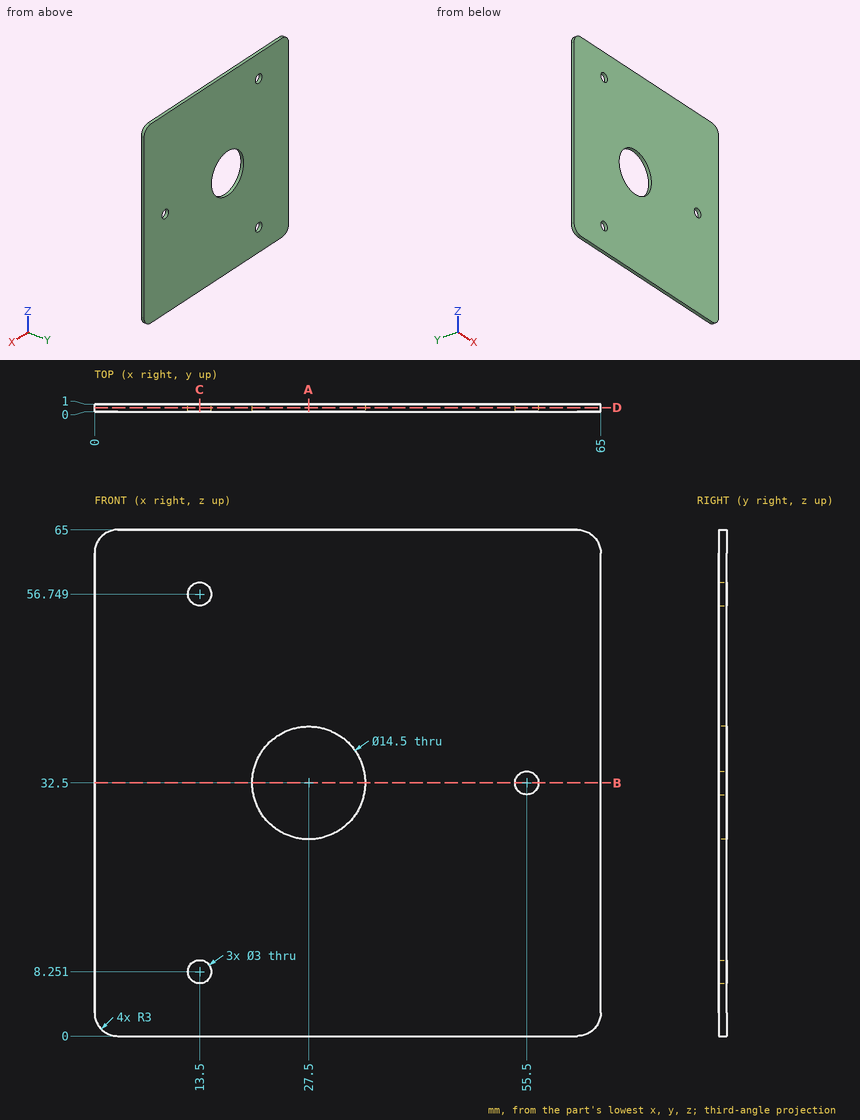
Geometry check sheet. Reference: drawing and pictorial views, mm from the part's lowest x, y, z. Give positions to 0.01 mm unless a question says otherwise; leave off trailing zeros. Loops run counter-clockwise (first coordinate to the right, second up) from the corner with the lowest first, then second, coordinate; pieces in that order, holes last. Notation, with made-up numbers: (-17, 46.5) - (-7, 46.5) arc R15 ccw to (-7, 74.5) - close; hole circle Ø5 at (28.5, -20.75). An arc over 180 degrees is marked (long way). Use CSV: the item, a comma, the result in double quotes. Start each with the question number.
Q1. Section check D-D, the plane y = 0.55. Record the cut outline in (x, z).
Q2. Section check C-C, the plane x = 13.5. Record the cut outline in (y, z).
Q3. Section check B-B, the plane z = 32.5. Record the cut outline in (x, y).
Q4. Scan lines: probe 1 along Z at (x, y) = (27, 0.4); probe 2 along X at (y, z) = (0.7, 33) (1 decimal); probe 3 along Z at (x, y) = (32, 0.65) (1 decimal). Record each from-to range of solid material in increasing order. Write a range as from..to.
Q5. Section check A-A, the plane x = 27.5. Record the cut outline in (y, z).
Q6. Go/stop test with a flat-tipped pin: pin 1 Ø8.5 at (x, z) = (27.5, 32.5) entering from -Y. Record where the tip stops, or that it passes through.
Findings below:
1,outline,"(0, 3) arc R3 ccw to (3, 0) - (62, 0) arc R3 ccw to (65, 3) - (65, 62) arc R3 ccw to (62, 65) - (3, 65) arc R3 ccw to (0, 62) - close; hole circle Ø3 at (13.5, 8.25); hole circle Ø3 at (13.5, 56.75); hole circle Ø14.5 at (27.5, 32.5); hole circle Ø3 at (55.5, 32.5)"
2,outline,"(0, 0) - (1, 0) - (1, 6.75) - (0, 6.75) - close; (0, 9.75) - (1, 9.75) - (1, 55.25) - (0, 55.25) - close; (0, 58.25) - (1, 58.25) - (1, 65) - (0, 65) - close"
3,outline,"(0, 0) - (20.25, 0) - (20.25, 1) - (0, 1) - close; (34.75, 0) - (54, 0) - (54, 1) - (34.75, 1) - close; (57, 0) - (65, 0) - (65, 1) - (57, 1) - close"
4,probe 1,"z = 0..25.27, 39.73..65"
4,probe 2,"x = 0..20.3, 34.7..54.1, 56.9..65"
4,probe 3,"z = 0..26.8, 38.2..65"
5,outline,"(0, 0) - (1, 0) - (1, 25.25) - (0, 25.25) - close; (0, 39.75) - (1, 39.75) - (1, 65) - (0, 65) - close"
6,pin 1,"passes through"
